Model file for the job. Use its own axes, mm. A direction names the side the tool comes from. Round coordinates to 2 decimals unless told otherwise and drop trailing zeros. Order: outer loops, then holes, each group sorted by start corner. A loop starts at its lowest first (then second) coordinate and runs counter-clockwise, first axis right, second up. Notation, with made-up numbers: (7.25, 38.5) -> (23.25, 38.5) arc R19 ccw to (23.25, 49.5) -> close; hole circle Ø6 at (6, 37). An arc over 180 degrees is marked (long way). Answer as CSV lines item,"result".
```python
from build123d import *

# Parameters (mm, degrees)
SKETCH1_R               = 33
SKETCH1_R_2             = 1.25
SKETCH1_R_3             = 1
BOSS_EXTRUDE2_DEPTH     = 2.5
CUT_EXTRUDE1_DEPTH      = 3.5
CUT_EXTRUDE1_DEPTH_BACK = 10
CHAMFER5_SIZE           = 0.25


with BuildPart() as part:
    # Sketch1 → Boss-Extrude2 (new body)
    with BuildSketch(Plane(origin=(0, 0, 0), x_dir=(1, 0, 0), z_dir=(0, 1, 0))):
        Circle(SKETCH1_R)
        with Locations((0, 27.5)):
            Circle(SKETCH1_R_2, mode=Mode.SUBTRACT)
        with Locations((27.5, 0)):
            Circle(SKETCH1_R_2, mode=Mode.SUBTRACT)
        with Locations((0, -27.5)):
            Circle(SKETCH1_R_2, mode=Mode.SUBTRACT)
        with Locations((-27.5, 0)):
            Circle(SKETCH1_R_2, mode=Mode.SUBTRACT)
        Circle(SKETCH1_R_3, mode=Mode.SUBTRACT)
    extrude(amount=BOSS_EXTRUDE2_DEPTH)

    # Sketch2 → Cut-Extrude1 (cut, two sides)
    with BuildSketch(Plane(origin=(0, 0, 0), x_dir=(1, 0, 0), z_dir=(0, 1, 0))) as cut_extrude1_sk:
        with BuildLine():
            ThreePointArc((25, 0), (0, 25), (-25, 0))
            ThreePointArc((-25, 0), (-20, -5), (-15, 0))
            ThreePointArc((-15, 0), (0, 15), (15, 0))
            ThreePointArc((15, 0), (20, -5), (25, 0))
        make_face()
    extrude(amount=CUT_EXTRUDE1_DEPTH, mode=Mode.SUBTRACT)
    extrude(cut_extrude1_sk.sketch, amount=-CUT_EXTRUDE1_DEPTH_BACK, mode=Mode.SUBTRACT)

    # Chamfer5
    chamfer5_edges = [part.edges().sort_by_distance(p)[0] for p in [
        (-1, 2.5, 0),
    ]]
    chamfer(chamfer5_edges, length=CHAMFER5_SIZE)


solid = part.part
```
Q1. Flat gauge pins, fed straight in: pin 1 (1.5 mm diameter, centred on x = -13, y = 1.5, fed in from +Z); pin 2 (1 mm diameter, centred on y = 1, z = 22.5, fed in from +X); pin 3 (1.5 mm diameter, centred on y = 2, z = -5.5, fed in from -X). Where does each tip first touch, or does it go through?
Checks:
pin 1,"z = 30.64"
pin 2,"x = 24.6"
pin 3,"x = -32.66"
Q2. Saw through at B-B (y = 0.45). Write the cut outline in (x, z).
Checks:
outline,"circle Ø66 at (0, 0); hole circle Ø2.5 at (-27.5, 0); hole (-25, 0) arc R25 ccw to (25, 0) arc R5 ccw to (15, 0) arc R15 cw to (-15, 0) arc R5 ccw to start; hole circle Ø2.5 at (0, -27.5); hole circle Ø2.5 at (0, 27.5); hole circle Ø2 at (0, 0); hole circle Ø2.5 at (27.5, 0)"
Q3. Wall check: L1, parallel to Z at x = 0, y = 1.1; L2, parallel to X at y = 1.75, z = -12.5; L3, parallel to X at y = 0.95, z = -11. Give the ranges that are in metal, low to high. Write a range as [from, to].
Checks:
L1,"[-33, -28.75], [-26.25, -25], [-15, -1], [1, 26.25], [28.75, 33]"
L2,"[-30.54, -21.65], [-8.29, 8.29], [21.65, 30.54]"
L3,"[-31.11, -22.45], [-10.2, 10.2], [22.45, 31.11]"
Q4. Mould opens along X. For faces 3 (the cylindrical face through (0, 1, -15)), 4 (the cylindrical face through (30.5, 1.2, 12.6)), 5 (the flat face through (0, 2.5, 7)) say: +X half, -X half, draft (parallel to the pull), parting line (faces both ways), or undercut.
Checks:
face 3,"undercut"
face 4,"parting line"
face 5,"draft"
Q5. Saw through at A-A (x = -11.5). Write the cut outline in (y, z), plus the area to 3 significant figures.
Checks:
outline,"(0, -30.93) -> (2.5, -30.93) -> (2.5, -22.2) -> (0, -22.2) -> close; (0, -9.63) -> (2.5, -9.63) -> (2.5, 30.93) -> (0, 30.93) -> close"
area,"123 mm²"
Q6. Saw through at D-D (z = 27.5). Write the cut outline in (x, y), plus the area to 3 significant figures.
Checks:
outline,"(-18.24, 0) -> (-1.25, 0) -> (-1.25, 2.5) -> (-18.24, 2.5) -> close; (1.25, 0) -> (18.24, 0) -> (18.24, 2.5) -> (1.25, 2.5) -> close"
area,"85.0 mm²"
Q7. Saw through at C-C (x = 0). Write the cut outline in (y, z), plus the area to 3 significant figures.
Checks:
outline,"(0, -33) -> (2.5, -33) -> (2.5, -28.75) -> (0, -28.75) -> close; (0, -26.25) -> (2.5, -26.25) -> (2.5, -25) -> (0, -25) -> close; (0, -15) -> (2.5, -15) -> (2.5, -1.25) -> (2.25, -1) -> (0, -1) -> close; (0, 1) -> (2.25, 1) -> (2.5, 1.25) -> (2.5, 26.25) -> (0, 26.25) -> close; (0, 28.75) -> (2.5, 28.75) -> (2.5, 33) -> (0, 33) -> close"
area,"122 mm²"
Q8. Tool access for faces 1 (the flat face through (0, 0, 7)), 2 (the cylindrical face through (20, 1, 5)): list every direction of +Z, -Z, +X, -X, +Y, -Y with a clear straight run to the whole face (end or side of a thin tool).
Checks:
face 1,"+Z, -Z, +X, -X, -Y"
face 2,"+Y, -Y"
